```python
from build123d import *

# Parameters (mm, degrees)
F1_DEPTH = 12.7
F2_R     = 5.08
F3_R     = 2.54
F4_R     = 1.27


with BuildPart() as f1:
    # F0 (on Front) → F1 (new body)
    with BuildSketch(Plane.XZ):
        Polygon((7.609934, 0), (0, 0), (0, 5.08), (-5.08, 5.08), (-5.08, -16.51), (61.221046, -16.51), (61.221046, 5.08), (61.221046, 36.83), (175.521046, 36.83), (175.521046, 57.15), (171.711046, 57.15), (171.711046, 52.07), (61.221046, 52.07), (61.221046, 57.15), (43.441046, 57.15), (43.441046, 5.08), (7.609934, 5.08), align=None)
    extrude(amount=F1_DEPTH)

    # F2
    f2_edges = [f1.edges().sort_by_distance(p)[0] for p in [
        (61.221046, -6.35, -16.51),
        (43.441046, -6.35, 57.15),
        (43.441046, -6.35, 5.08),
        (61.221046, -6.35, 36.83),
        (175.521046, -6.35, 36.83),
        (-5.08, -6.35, -16.51),
    ]]
    fillet(f2_edges, radius=F2_R)

    # F3
    f3_edges = [f1.edges().sort_by_distance(p)[0] for p in [
        (116.466046, -12.7, 52.07),
        (116.466046, 0, 52.07),
    ]]
    fillet(f3_edges, radius=F3_R)

    # F4
    f4_edges = [f1.edges().sort_by_distance(p)[0] for p in [
        (43.441046, -12.7, 31.115),
        (22.98549, 0, 5.08),
        (-5.08, -12.7, -3.175),
        (-5.08, 0, -3.175),
        (61.221046, -6.35, 57.15),
        (171.711046, -6.35, 57.15),
        (175.521046, -6.35, 57.15),
    ]]
    fillet(f4_edges, radius=F4_R)


solid = f1.part
```
Input: part model. Units: mm. Frame: model coordinates. A direction names the side the tool comes from. Round coordinates to 2 decimals unless told otherwise and drop trailing zeros. Loops run counter-clockwise (first coordinate to the right, second up) from the corner with the lowest first, then second, coordinate; pieces in that order, holes last. Notation, with made-up numbers: (20, 20) - (75, 20) arc R4 ccw to (75, 24) - close; hole circle Ø8 at (-16.5, 46.25). An arc over 180 degrees is marked (long way). One line per item, written item: value. Start each with the question number.
(1) Section B-B, the plane y = -7.5. Return loops of the section in (x, z), plus the area to 3 significant figures.
(2) Ray query, line 1 (Z direction, x = 86, y = -3); line 2 (Z direction, x = 37, y = -2.25); line 3 (X direction, y = -6.75, z = 49). Return the intervals inside material, ascending. Write a range as [from, to].
(3) Section C-C, the plane x = 18.5. Return loops of the section in (y, z).
(4) Contact query for flat-ended pins moving along their axis: P1, Ø4, axis at y = -3, z = 29.5, coming from the -X side; P2, Ø2.5, axis at x = -1.5, y = -6.5, coming from the +Z side; P3, Ø1.5, axis at y = -5, z = 3.5, coming from the +X side. Output: stop coordinate, or through.
(5) Access query for faces 4 (the flat face through (118, -6, 36.83)), 5 (the flat face through (-5.08, -6, -3)), 6 (the flat face through (43.441, -6, 31)), 7 (the flat face through (117, -6, 52.07)). Directions: +Z, -Z, +X, -X, +Y, -Y. A direction counts if a zero-diameter tool reaches every point of the face in a straight line with its end or side. Return the directions, or none.
(6) Draft query along X for faces 1 (the cylindrical face through (44.97, -6.42, 55.7)), 2 (the flat face through (58, -12.7, 24)), 3 (the flat face through (4, -6, 0)). Return one class per face: +X half, -X half, draft (parallel to the pull), parting line (faces both ways), or undercut.
(7) Section A-A, the plane z = 24.5. Return loops of the section in (x, y).
Results below:
1. outline: (-5.08, -11.43) arc R5.08 ccw to (0, -16.51) - (56.14, -16.51) arc R5.08 ccw to (61.22, -11.43) - (61.22, 31.75) arc R5.08 cw to (66.3, 36.83) - (170.44, 36.83) arc R5.08 ccw to (175.52, 41.91) - (175.52, 55.88) arc R1.27 ccw to (174.25, 57.15) - (172.98, 57.15) arc R1.27 ccw to (171.71, 55.88) - (171.71, 52.07) - (61.22, 52.07) - (61.22, 55.88) arc R1.27 ccw to (59.95, 57.15) - (48.52, 57.15) arc R5.08 ccw to (43.44, 52.07) - (43.44, 10.16) arc R5.08 cw to (38.36, 5.08) - (7.61, 5.08) - (7.61, 0) - (0, 0) - (0, 5.08) - (-5.08, 5.08) - close
1. area: 4,070 mm^2
2. line 1: [36.83, 52.07]
2. line 2: [-16.51, 5.08]
2. line 3: [43.44, 175.52]
3. outline: (-12.7, -15.24) arc R1.27 ccw to (-11.43, -16.51) - (-1.27, -16.51) arc R1.27 ccw to (0, -15.24) - (0, 3.81) arc R1.27 ccw to (-1.27, 5.08) - (-11.43, 5.08) arc R1.27 ccw to (-12.7, 3.81) - close
4. P1: x = 43.44
4. P2: z = 5.08
4. P3: x = 61.22
5. face 4: -Z, +X, +Y, -Y
5. face 5: +Z, -Z, -X, +Y, -Y
5. face 6: +Z, -X, +Y, -Y
5. face 7: +Z, +Y, -Y
6. face 1: -X half
6. face 2: draft
6. face 3: undercut
7. outline: (43.44, -11.43) arc R1.27 ccw to (44.71, -12.7) - (59.95, -12.7) arc R1.27 ccw to (61.22, -11.43) - (61.22, -1.27) arc R1.27 ccw to (59.95, 0) - (44.71, 0) arc R1.27 ccw to (43.44, -1.27) - close
